```python
from build123d import *

# Parameters (mm, degrees)
SKETCH1_R           = 3.175
BOSS_EXTRUDE1_DEPTH = 4.7625
SKETCH2_W           = 4.7625
SKETCH2_H           = 33.783
CUT_EXTRUDE1_DEPTH  = 5


with BuildPart() as part:
    # Sketch1 → Boss-Extrude1 (new body)
    with BuildSketch(Plane(origin=(0, 0, 0), x_dir=(1, 0, 0), z_dir=(0, 1, 0))):
        with BuildLine():
            Line((-82.674132744, 104.451069294), (-69.310188895, 104.451069294))
            ThreePointArc((-69.310188895, 104.451069294), (-55.336180049, 99.157726681), (-42.113057451, 106.117714323))
            Line((-42.113057451, 106.117714323), (0, 94.833554589))
            Line((0, 94.833554589), (0, 58.293))
            Line((0, 58.293), (8, 58.293))
            Line((8, 58.293), (8, -58.293))
            Line((8, -58.293), (0, -58.293))
            Line((0, -58.293), (0, -94.833554589))
            Line((0, -94.833554589), (-42.113057451, -106.117714323))
            ThreePointArc((-42.113057451, -106.117714323), (-55.336180049, -99.157726681), (-69.310188895, -104.451069294))
            Line((-69.310188895, -104.451069294), (-82.674132744, -104.451069294))
            ThreePointArc((-82.674132744, -104.451069294), (-86.841727728, -94.209575285), (-83.629476528, -83.629476528))
            Line((-83.629476528, -83.629476528), (0, 0))
            Line((0, 0), (-83.629476528, 83.629476528))
            ThreePointArc((-83.629476528, 83.629476528), (-86.841727728, 94.209575285), (-82.674132744, 104.451069294))
        make_face()
        with Locations((-70.310188895, 93.451069294)):
            Circle(SKETCH1_R, mode=Mode.SUBTRACT)
        with Locations((-70.310188895, -93.451069294)):
            Circle(SKETCH1_R, mode=Mode.SUBTRACT)
    extrude(amount=BOSS_EXTRUDE1_DEPTH)

    # Sketch2 → Cut-Extrude1 (cut)
    with BuildSketch(Plane(origin=(0, 0, 0), x_dir=(1, 0, 0), z_dir=(0, 1, 0))):
        Polygon((-17.19282542, -99.440358276), (-4.829629131, -96.127649814), (-6.062254834, -91.527428067), (-18.425451123, -94.840136528), align=None)
        Polygon((-37.283428319, -104.823619098), (-24.920232031, -101.510910637), (-26.152857733, -96.910688889), (-38.516054022, -100.22339735), align=None)
        with Locations((5.61875, -33.4015)):
            Rectangle(SKETCH2_W, SKETCH2_H)
        Polygon((-38.516054022, 100.22339735), (-26.152857733, 96.910688889), (-24.920232031, 101.510910637), (-37.283428319, 104.823619098), align=None)
        Polygon((-18.425451123, 94.840136528), (-6.062254834, 91.527428067), (-4.829629131, 96.127649814), (-17.19282542, 99.440358276), align=None)
        with Locations((5.61875, 33.4015)):
            Rectangle(SKETCH2_W, SKETCH2_H)
    extrude(amount=CUT_EXTRUDE1_DEPTH, mode=Mode.SUBTRACT)


solid = part.part
```
The model under review builds one solid part; all positions refer to its coordinate system, in mm. A direction names the side the tool comes from. Coordinates: 2 decimals unless noted, no trailing zeros. Write each loop counter-clockwise with the first axis right and the second up, starting at its lowest first coordinate (ties: lowest second). Pieces come first, ordered by that corner, then holes. Notation, with made-up numbers: (-3, 36.25) -> (8, 36.25) arc R19 cw to (8, 65.25) -> close; hole circle Ø10 at (-33, 41.5). An arc over 180 degrees is marked (long way). One line per item, written item: value. Start each with the question number.
Q1. Add section C-C, the plane x = -30.5. Give the boundary of the cut face in (y, z).
Q2. Clearance check with flat-ended pins moving along their axes: P1, Ø1.4, axis at x = 3.5, y = 2, coming from the +Z side; P2, Ø2.5, axis at x = -77, y = 2.5, coming from the +Z side; P3, Ø2.5, axis at x = -73, y = 2, coming from the -Z side. State where each tip first meets the part, or that it passes through.
Q3. Add section D-D, the plane y = 1.95. Count the separate pieces of the cut face and the enclosed holes in it, then the cut area to 3 significant figures.
Q4. For faces 4 (the face through (-17.818, 2.348, 97.108)), 5 (the face through (-25.53, 2.35, 99.24)), 6 (the face through (-76, 2, -104.451)), 7 (the face through (6, 2, -16.51)), list the 3-axis set-ups (+Z, -Z, +X, -X, +Y, -Y) from which the entire face can be reached by the end or side of a thin tool; tool diameter is ignored.
Q5. The part is to be moulded in two halves that separate along X. For faces 1 (the face through (-86.85, 2.35, -94.05)), 2 (the face through (0, 2, 76)), 3 (the face through (-68.85, 2.35, 96.27)), say which applies: +X half, -X half, draft (parallel to the pull), parting line (faces both ways), or undercut.
Q6. Add section B-B, the plane z = 62.5. Give the boundary of the cut face in (x, y), then the cut area to 3 significant figures.
Q7. Add section A-A, the plane x = -78. Give the boundary of the cut face in (y, z).
Q8. To check wall thickness, follow probe 1 along Z at (x, y) = (-72, 3.5); probe 2 along Z at (x, y) = (1, 2.45); probe 3 along Z at (x, y) = (-13, 3.25). State the ranges of each line that lie inside material, in increasing order.
Response:
1. outline: (0, -98.08) -> (4.76, -98.08) -> (4.76, -30.5) -> (0, -30.5) -> close; (0, 30.5) -> (4.76, 30.5) -> (4.76, 98.08) -> (0, 98.08) -> close
2. P1: z = 58.29
2. P2: z = 104.45
2. P3: z = -104.45
3. separate pieces: 1
3. enclosed holes: 2
3. area: 10,300 mm²
4. face 4: +Y, -Y
4. face 5: +Z, +Y, -Y
4. face 6: -Z, -X, +Y, -Y
4. face 7: +X, +Y, -Y
5. face 1: -X half
5. face 2: +X half
5. face 3: undercut
6. outline: (-62.5, 0) -> (0, 0) -> (0, 4.76) -> (-62.5, 4.76) -> close
6. area: 298 mm²
7. outline: (0, -104.45) -> (4.76, -104.45) -> (4.76, -78) -> (0, -78) -> close; (0, 78) -> (4.76, 78) -> (4.76, 104.45) -> (0, 104.45) -> close
8. probe 1: -104.45 to -96.14, -90.76 to -72, 72 to 90.76, 96.14 to 104.45
8. probe 2: -58.29 to 58.29
8. probe 3: -93.39 to -13, 13 to 93.39
